Check sheet for the drawn part. Datum: minimum x, y, z corner. Units: mm. Coordinates: 2 decimals unless noted, no trailing zeros. Write each loop counter-clockwise with the first axis right and the second up, starting at its lowest first coordinate (ties: lowest second). Pieces come first, ordered by that corner, then holes. Notation, with made-up numbers: (-29.75, 29.5) - (-0.75, 29.5) arc R17 cw to (-0.75, 38.5) - close; hole circle Ø8 at (36, -20). An arc over 180 degrees is marked (long way). Write each question's results on one line, items separated by ' | '.
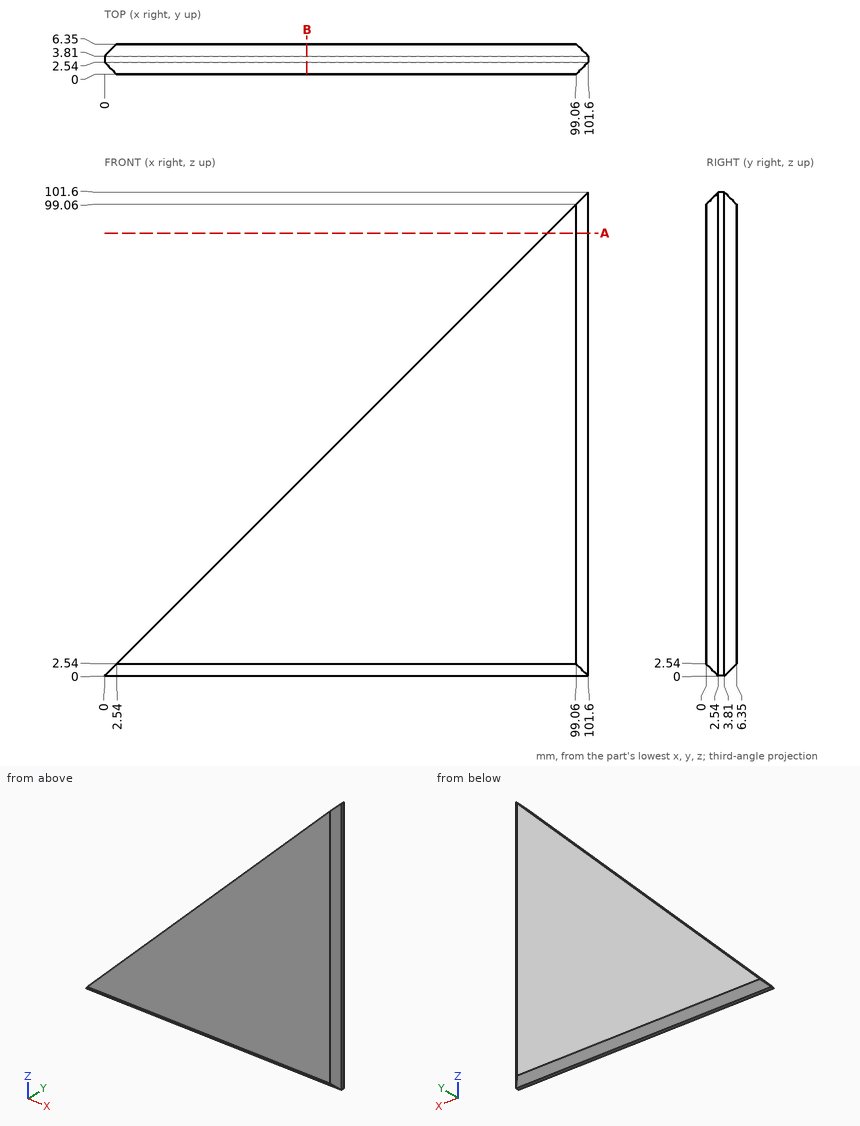
1. Material ranges on L1, parallel to X at y = 1.25, z = 96.5; L2, parallel to Z at x = 52.5, y = 3.5; L3, parallel to X at y = 6, z = 67.5, recorded low to high. Write a range as [from, to].
Values follow:
L1: x = [96.5, 100.31] | L2: z = [0, 52.5] | L3: x = [67.5, 99.41]
2. Sectioned sample at B-B (x = 42.5). Record the cut outline in (y, z), then the cut area to 3 significant figures.
Values follow:
outline: (0, 2.54) - (2.54, 0) - (3.81, 0) - (6.35, 2.54) - (6.35, 42.5) - (0, 42.5) - close | area: 263 mm^2
3. Go/stop test with flat-tipped pins: pin 1 (3 mm diameter, centred on x = 67, y = 0.5, fed in from +Z); pin 2 (3 mm diameter, centred on y = 4, z = 34, fed in from -X). Record where each tip stops, or that it passes through.
Values follow:
pin 1: stops at z = 68.5 | pin 2: stops at x = 32.5
4. Sectioned sample at A-A (z = 93). Record the cut outline in (x, y).
Values follow:
outline: (93, 0) - (99.06, 0) - (101.6, 2.54) - (101.6, 3.81) - (99.06, 6.35) - (93, 6.35) - close
